```python
from build123d import *

# Parameters (mm, degrees)
BOSS_EXTRUDE1_DEPTH      = 3.175
SKETCH2_R                = 16.9545
CUT_EXTRUDE1_DEPTH       = 600.06621556
FILLET1_R                = 15.875
CONVERT_SOLID1_START     = -1.5875
CONVERT_SOLID1_OUTLINE_R = 16.9545
CONVERT_SOLID1_DEPTH     = 1.5875
EDGE_FLANGE1_START       = 76.99375
EDGE_FLANGE1_DEPTH       = 240.50625
EDGE_FLANGE1_START_2     = 79.375
EDGE_FLANGE1_2_DEPTH     = 238.125
EDGE_FLANGE1_START_3     = -3
EDGE_FLANGE1_3_DEPTH     = 9.35
FILLET2_R                = 25.4
FILLET3_R                = 3.175
CUT_EXTRUDE2_DEPTH       = 4.7625
FILLET4_R                = 3.175
EDGE_FLANGE3_DEPTH       = 341.057724741
FILLET5_R                = 9.525
CUT_EXTRUDE3_DEPTH       = 4.7625
FILLET7_R                = 12.7
SKETCH17_R               = 3.302
CUT_EXTRUDE4_DEPTH       = 608.612384802
CUT_EXTRUDE5_DEPTH       = 608.612384802
SKETCH19_R               = 3.302
CUT_EXTRUDE6_DEPTH       = 533.561746786


with BuildPart() as part:
    # Sketch1 → Boss-Extrude1 (new body)
    with BuildSketch(Plane.XY):
        with BuildLine():
            Line((6.35, 0), (317.5, 0))
            Line((317.5, 0), (317.5, 25.4))
            Line((317.5, 25.4), (181.457249023, 52.608550195))
            ThreePointArc((181.457249023, 52.608550195), (140.315142877, 75.746018143), (120.694108864, 118.676547437))
            Line((120.694108864, 118.676547437), (76.2, 508))
            Line((76.2, 508), (6.35, 508))
            ThreePointArc((6.35, 508), (1.859871939, 506.140128061), (0, 501.65))
            Line((0, 501.65), (0, 6.35))
            ThreePointArc((0, 6.35), (1.859871939, 1.859871939), (6.35, 0))
        make_face()
    extrude(amount=BOSS_EXTRUDE1_DEPTH)

    # Sketch2 → Cut-Extrude1 (cut, through all)
    with BuildSketch(Plane.XY.offset(3.175)):
        with Locations((20.574, 486.9942)):
            Circle(SKETCH2_R)
        with Locations((20.574, 20.574)):
            Circle(SKETCH2_R)
    extrude(amount=-CUT_EXTRUDE1_DEPTH, mode=Mode.SUBTRACT)

    # Fillet1
    fillet1_edges = [part.edges().sort_by_distance(p)[0] for p in [
        (317.5, 25.4, 1.5875),
    ]]
    fillet(fillet1_edges, radius=FILLET1_R)

    # Convert-Solid1: read off the stored shape, not the designer's step
    # Convert-Solid1 outline → Convert-Solid1 (add)
    with BuildSketch(Plane.XY.offset(CONVERT_SOLID1_START)):
        with BuildLine():
            Line((304.738343645, 27.952331271), (181.457249023, 52.608550195))
            ThreePointArc((181.457249023, 52.608550195), (140.315142877, 75.746018143), (120.694108864, 118.676547437))
            Line((120.694108864, 118.676547437), (76.2, 508))
            Line((76.2, 508), (6.35, 508))
            ThreePointArc((6.35, 508), (1.859871939, 506.140128061), (0, 501.65))
            Line((0, 501.65), (0, 6.35))
            ThreePointArc((0, 6.35), (1.859871939, 1.859871939), (6.35, 0))
            Line((6.35, 0), (317.5, 0))
            Line((317.5, 0), (317.5, 12.385613044))
            ThreePointArc((317.5, 12.385613044), (313.901806494, 22.450186921), (304.738343645, 27.952331271))
        make_face()
        with Locations((20.574, 20.574)):
            Circle(CONVERT_SOLID1_OUTLINE_R, mode=Mode.SUBTRACT)
        with Locations((20.574, 486.9942)):
            Circle(CONVERT_SOLID1_OUTLINE_R, mode=Mode.SUBTRACT)
    extrude(amount=CONVERT_SOLID1_DEPTH)

    # Edge-Flange1: read off the stored shape, not the designer's step
    # Edge-Flange1 outline → Edge-Flange1 (cut)
    with BuildSketch(Plane.YZ.offset(EDGE_FLANGE1_START)):
        with BuildLine():
            ThreePointArc((7.9375, -1.5875), (3.589952199, -0.290988961), (0.662661084, 3.175))
            Line((0.662661084, 3.175), (0, 3.175))
            Line((0, 3.175), (0, -1.5875))
            Line((0, -1.5875), (7.9375, -1.5875))
        make_face()
    extrude(amount=EDGE_FLANGE1_DEPTH, mode=Mode.SUBTRACT)

    # Edge-Flange1 2 outline → Edge-Flange1 2 (add)
    with BuildSketch(Plane.YZ.offset(EDGE_FLANGE1_START_2)):
        with BuildLine():
            Line((0, 104.775), (0, 6.35))
            ThreePointArc((0, 6.35), (0.167431141, 4.728292203), (0.662661084, 3.175))
            Line((0.662661084, 3.175), (7.9375, 3.175))
            ThreePointArc((7.9375, 3.175), (5.69243597, 4.10493597), (4.7625, 6.35))
            Line((4.7625, 6.35), (4.7625, 104.775))
            Line((4.7625, 104.775), (0, 104.775))
        make_face()
    extrude(amount=EDGE_FLANGE1_2_DEPTH)

    # Edge-Flange1 3 outline → Edge-Flange1 3 (cut)
    with BuildSketch(Plane.XY.offset(EDGE_FLANGE1_START_3)):
        with BuildLine():
            Line((79.375, -1), (79.375, 10.31875))
            ThreePointArc((79.375, 10.31875), (78.184375, 11.509375), (76.99375, 10.31875))
            Line((76.99375, 10.31875), (76.99375, -1))
            Line((76.99375, -1), (79.375, -1))
        make_face()
    extrude(amount=EDGE_FLANGE1_3_DEPTH, mode=Mode.SUBTRACT)

    # Fillet2
    fillet2_edges = [part.edges().sort_by_distance(p)[0] for p in [
        (79.375, 2.38125, 104.775),
        (317.5, 2.38125, 104.775),
    ]]
    fillet(fillet2_edges, radius=FILLET2_R)

    # Fillet3
    fillet3_edges = [part.edges().sort_by_distance(p)[0] for p in [
        (76.99375, 0, 0.79375),
    ]]
    fillet(fillet3_edges, radius=FILLET3_R)

    # Sketch7 → Cut-Extrude2 (cut)
    with BuildSketch(Plane.XY.offset(3.175)):
        with BuildLine():
            Line((24.053808826, 405.037372989), (60.983957397, 81.898572989))
            ThreePointArc((60.983957397, 81.898572989), (55.486376009, 64.57864546), (38.902693748, 57.15))
            Line((38.902693748, 57.15), (0, 57.15))
            Line((0, 57.15), (0, 424.7388))
            Line((0, 424.7388), (1.972545176, 424.7388))
            ThreePointArc((1.972545176, 424.7388), (16.768899716, 419.097482261), (24.053808826, 405.037372989))
        make_face()
    extrude(amount=-CUT_EXTRUDE2_DEPTH, mode=Mode.SUBTRACT)

    # Fillet4
    fillet4_edges = [part.edges().sort_by_distance(p)[0] for p in [
        (0, 424.7388, 0.79375),
        (0, 57.15, 0.79375),
    ]]
    fillet(fillet4_edges, radius=FILLET4_R)

    # Edge-Flange3: sheet metal written as solids
    # Edge-Flange3 section (on a plane across the edge) → Edge-Flange3 (add)
    with BuildSketch(Plane(origin=(125.425808218, 119.217313077, 3.175), x_dir=(-0.9935326726564042, -0.11354659116073179, 3.4914813388431334e-15), z_dir=(-0.11354659116073179, 0.9935326726564042, 0))):
        with BuildLine():
            Line((-4.7625, 4.7625), (-4.7625, 46.0375))
            Line((-4.7625, 46.0375), (0, 46.0375))
            Line((0, 46.0375), (0, 4.7625))
            ThreePointArc((0, 4.7625), (1.394903955, 1.394903955), (4.7625, 0))
            Line((4.7625, 0), (4.7625, -4.7625))
            ThreePointArc((4.7625, -4.7625), (-1.972692091, -1.972692091), (-4.7625, 4.7625))
        make_face()
    extrude(amount=EDGE_FLANGE3_DEPTH)

    # Fillet5
    fillet5_edges = [part.edges().sort_by_distance(p)[0] for p in [
        (127.791657895, 119.487695897, 49.2125),
        (89.065715861, 458.33968869, 49.2125),
    ]]
    fillet(fillet5_edges, radius=FILLET5_R)

    # Sketch16 → Cut-Extrude3 (cut)
    with BuildSketch(Plane.XY.offset(3.175)):
        Polygon((76.2, 508), (41.275, 508), (41.275, 457.528540229), (81.968166831, 457.528540229), align=None)
    extrude(amount=-CUT_EXTRUDE3_DEPTH, mode=Mode.SUBTRACT)

    # Fillet7
    fillet7_edges = [part.edges().sort_by_distance(p)[0] for p in [
        (41.275, 457.528540229, 0.79375),
        (41.275, 508, 0.79375),
    ]]
    fillet(fillet7_edges, radius=FILLET7_R)

    # Sketch17 → Cut-Extrude4 (cut, through all)
    with BuildSketch(Plane.XY.offset(3.175)):
        with Locations((76.2, 423.892006342)):
            Circle(SKETCH17_R)
        with Locations((76.2, 347.692006342)):
            Circle(SKETCH17_R)
        with Locations((76.2, 271.492006342)):
            Circle(SKETCH17_R)
        with Locations((76.2, 195.292006342)):
            Circle(SKETCH17_R)
        with Locations((76.2, 119.092006342)):
            Circle(SKETCH17_R)
        with Locations((266.7, 22.225)):
            Circle(SKETCH17_R)
        with Locations((165.1, 22.225)):
            Circle(SKETCH17_R)
    extrude(amount=-CUT_EXTRUDE4_DEPTH, mode=Mode.SUBTRACT)

    # Sketch18 → Cut-Extrude5 (cut, through all)
    with BuildSketch(Plane.XY.offset(3.175)):
        with BuildLine():
            Line((3.6195, 28.2067), (3.6195, 20.574))
            ThreePointArc((3.6195, 20.574), (20.574, 3.6195), (37.5285, 20.574))
            Line((37.5285, 20.574), (37.5285, 28.2067))
            ThreePointArc((37.5285, 28.2067), (20.574, 45.1612), (3.6195, 28.2067))
        make_face()
    extrude(amount=-CUT_EXTRUDE5_DEPTH, mode=Mode.SUBTRACT)

    # Sketch19 → Cut-Extrude6 (cut, through all)
    with BuildSketch(Plane(origin=(141.989587265, 16.227381402, 0), x_dir=(0, 0, -1), z_dir=(0.9935326726564043, 0.1135465911607318, -3.62817709114321e-15))):
        with Locations(Location((-28.575, 419.862347463, 0), (0, 0, 90))):
            Circle(SKETCH19_R)
        with Locations(Location((-28.575, 129.604622722, 0), (0, 0, 90))):
            Circle(SKETCH19_R)
    extrude(amount=-CUT_EXTRUDE6_DEPTH, mode=Mode.SUBTRACT)


solid = part.part
```
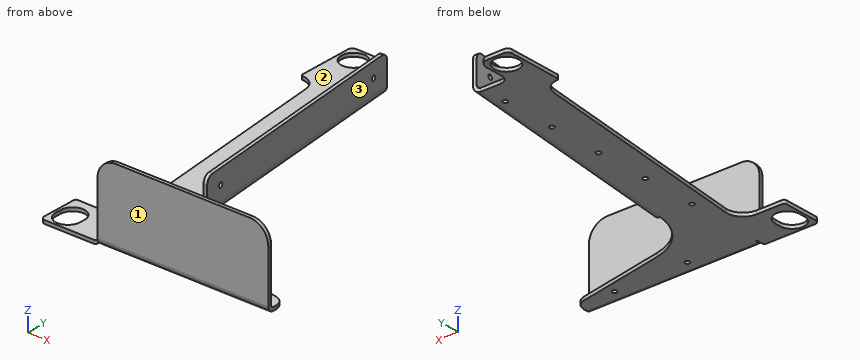
The model under review builds one solid part; all positions refer to its coordinate system, in mm. Face numbers are marked on the shaded views. Give positions to 0.01 mm unless a question says otherwise; leave off trailing zeros. Write each loop counter-clockwise with the first axis right and the second up, starting at its lowest first coordinate (ties: lowest second). Pieces come first, ordered by that corner, then holes. Notation, with made-up numbers: (14.25, 28.25) -> (19.25, 28.25) arc R20 ccw to (19.25, 37.25) -> close; hole circle Ø3 at (6, 53). An arc over 180 degrees is marked (long way). Put each result on its own line as item: value.
(1) We need section D-D, the plane y = 102.5. Give the boundary of the cut face in (x, z) (1 decimal).
Results are:
outline: (58.6, -1.6) -> (124.4, -1.6) -> (124.4, 3.2) -> (58.6, 3.2) -> close
(2) We need section C-C, the plane z = 56. Give the boundary of the cut face in (x, y) (1 decimal), and give its area (3 significant figures).
Results are:
outline: (79.4, 0) -> (317.5, 0) -> (317.5, 4.8) -> (79.4, 4.8) -> close
area: 1,130 mm²
(3) The part is to be moulded in two halves that separate along Y. For the marked faces 1, 2 and 3, say which applies: pulls with the +Y half, pulls with the -Y half, needs draft (parallel to the pull), parting line crosses it, or undercut.
Results are:
face 1: pulls with the -Y half
face 2: undercut
face 3: pulls with the +Y half
(4) For pin 1 Ø5 at (x, y) = (92.5, 102.5) entering from +Z (3 decimals); pin 2 Ø20.5 at (x, y) = (113, 265) entering from +Z; pin 3 Ø2.5 at (y, z) = (487.5, 0.5) entering from +X (3 decimals); pin 4 Ø7.5 at (x, y) = (76.2, 423.89) entering from -Z, all flat-tipped, find the tip position at first contact; note any pin that passes through.
Results are:
pin 1: z = 3.175
pin 2: z = 49.21
pin 3: x = 41.275
pin 4: z = -1.59
(5) We need section A-A, the plane y = 39.5. Give the boundary of the cut face in (x, z) (1 decimal), and give its area (3 significant figures).
Results are:
outline: (0, -1.6) -> (7.9, -1.6) -> (7.9, 3.2) -> (0, 3.2) -> close; (33.2, -1.6) -> (247, -1.6) -> (247, 3.2) -> (33.2, 3.2) -> close
area: 1,060 mm²
(6) To check wall thickness, follow probe 1 along Y at (x, z) = (76, 0); probe 2 along Y at (x, z) = (246.5, 80); probe 3 along Z at (x, y) = (89.5, 311) (1 decimal). State the ranges of each line that lie inside material, in increasing order. Write a range as from..to.
Results are:
probe 1: 0.87..115.8, 122.39..192, 198.59..268.2, 274.79..344.4, 350.99..420.6, 427.19..457.53
probe 2: 0..4.76
probe 3: -1.6..3.2
